Model file for the job. Use its own axes, mm. Give positions to 0.01 mm unless a question says otherwise; leave off trailing zeros. Order: outer loops, then holes, each group sorted by start corner. A loop starts at its lowest first (then second) coordinate and runs counter-clockwise, first axis right, second up. Notation, with made-up numbers: (15.25, -36) - (56.25, -36) arc R23 cw to (56.25, -13) - close; hole circle Ø7 at (52.25, -8.5). An arc over 180 degrees is marked (long way). Use CSV: the item, a comma, the result in double quotes. Start each with the question number.
(1) Pull direction X, two halves, no side cores. Call faces 1 (the cylindrical face through (9.76, -2.17, 5.07)), 2 (the cylindrical face through (0.28, 16.486, 104.297)), 3 (the flat face through (-20, 0, 56)): +X half, -X half, draft (parallel to the pull), parting line (faces both ways), or undercut.
(2) Band-saw the part on B-B, the plane y = -7. Give the cut face in (x, z).
(3) Drop a flat-ended pin along its axis: pin 1 Ø12 at (x, y) = (0, 0) entering from -Z. Give the stop position or say it passes through.
(4) Band-saw the part on D-D, the plane y = 15. Give the cut face in (x, z).
(5) Band-saw the part on A-A, the plane z = 18. Give the cut face in (x, y), then the cut area to 3 significant figures.
(6) Band-saw the part on C-C, the plane x = -5.5. Give the cut face in (y, z).
(7) Probe L1, parallel to X at y = 0, z = 6; L2, parallel to Y at x = 0, z = 5; L3, parallel to X at y = 8, z = 14. List the from-to ranges inside material, lowest first.
from build123d import *

# Parameters (mm, degrees)
F1_DEPTH = 20
F2_R     = 20


with BuildPart() as f1:
    # F0 (on Right) → F1 (new body, symmetric)
    with BuildSketch(Plane.YZ):
        with BuildLine():
            Line((-22.5, 0), (0, 0))
            Line((0, 0), (0, 85))
            ThreePointArc((0, 85), (-10, 95), (0, 105))
            Line((0, 105), (0, 110))
            Line((0, 110), (-22.5, 110))
            Line((-22.5, 110), (-22.5, 0))
        make_face()
        with BuildLine():
            Line((0, 0), (22.5, 0))
            Line((22.5, 0), (22.5, 110))
            Line((22.5, 110), (0, 110))
            Line((0, 110), (0, 105))
            ThreePointArc((0, 105), (7.0710678119, 102.0710678119), (10, 95))
            ThreePointArc((10, 95), (7.0710678119, 87.9289321881), (0, 85))
            Line((0, 85), (0, 0))
        make_face()
    extrude(amount=F1_DEPTH, both=True)

    # F2
    f2_edges = [f1.edges().sort_by_distance(p)[0] for p in [
        (0, -22.5, 110),
        (0, 22.5, 110),
    ]]
    fillet(f2_edges, radius=F2_R)

    # F3 (on Right) → F4 (revolve, cut)
    with BuildSketch(Plane.YZ):
        with BuildLine():
            Line((0, 20), (0, 0))
            Line((0, 0), (0, -5))
            Line((0, -5), (10, -5))
            Line((10, -5), (10, 0))
            Line((10, 0), (10, 10))
            ThreePointArc((10, 10), (7.0710678119, 17.0710678119), (0, 20))
        make_face()
    revolve(axis=Axis((0, 0, 10), (0, 0, 1)), mode=Mode.SUBTRACT)


solid = f1.part
Answer block:
1,face 1,"undercut"
1,face 2,"draft"
1,face 3,"-X half"
2,outline,"(-20, 0) - (-7.14, 0) - (-7.14, 10) arc R7.14 cw to (7.14, 10) - (7.14, 0) - (20, 0) - (20, 87.86) - (-20, 87.86) - close; (-20, 102.14) - (20, 102.14) - (20, 109.49) - (-20, 109.49) - close"
3,pin 1,"stops at z = 18"
4,outline,"(-20, 0) - (20, 0) - (20, 105.61) - (-20, 105.61) - close"
5,outline,"(-20, -22.5) - (20, -22.5) - (20, 22.5) - (-20, 22.5) - close; hole circle Ø12 at (0, 0)"
5,area,"1,690 mm2"
6,outline,"(-22.5, 0) - (-8.35, 0) - (-8.35, 10) arc R8.35 cw to (8.35, 10) - (8.35, 0) - (22.5, 0) - (22.5, 90) arc R20 ccw to (2.5, 110) - (-2.5, 110) arc R20 ccw to (-22.5, 90) - close; hole circle Ø20 at (0, 95)"
7,L1,"x = -20 to -10, 10 to 20"
7,L2,"y = -22.5 to -10, 10 to 22.5"
7,L3,"x = -20 to -4.47, 4.47 to 20"
